from build123d import *

# Parameters (mm, degrees)
BOSS_EXTRUDE1_DEPTH      = 37.5
BOSS_EXTRUDE1_DEPTH_BACK = 37.5
SKETCH1_W                = 20
SKETCH1_H                = 10
SKETCH3_W                = 20
SKETCH3_H                = 5
BOSS_EXTRUDE2_DEPTH      = 20
FILLET1_R                = 10
SKETCH5_W                = 20
SKETCH5_H                = 5
BOSS_EXTRUDE3_DEPTH      = 25
CHAMFER1_SIZE            = 5
CHAMFER1_SIZE_2          = 8.660254038
FILLET2_R                = 10
CUT_EXTRUDE1_DEPTH       = 65.08002809
CUT_EXTRUDE1_DEPTH_BACK  = 65.08002809
SKETCH4_R                = 2.75
CUT_EXTRUDE2_DEPTH       = 66.048059156
CUT_EXTRUDE2_DEPTH_BACK  = 2.5


# Some blends are built 0.0001 mm under size
with BuildPart() as part:
    # Sketch1 → Boss-Extrude1 (new, two sides: drawn at the far end of the back side and taken through both)
    with BuildSketch(Plane.XY.offset(-BOSS_EXTRUDE1_DEPTH_BACK)):
        Rectangle(SKETCH1_W, SKETCH1_H)
    extrude(amount=BOSS_EXTRUDE1_DEPTH + BOSS_EXTRUDE1_DEPTH_BACK)

    # Sketch3 → Boss-Extrude2 (add)
    with BuildSketch(Plane(origin=(0, 0, -37.5), x_dir=(-1, 0, 0), z_dir=(0, 0, -1))):
        Rectangle(SKETCH3_W, SKETCH3_H)
    extrude(amount=BOSS_EXTRUDE2_DEPTH)

    # Fillet1
    fillet1_edges = [part.edges().sort_by_distance(p)[0] for p in [
        (-10, 0, -57.5),
        (10, 0, -57.5),
    ]]
    fillet(fillet1_edges, radius=FILLET1_R - 0.0001)  # a hair under: the kernel refuses the full size

    # Sketch5 → Boss-Extrude3 (add)
    with BuildSketch(Plane.XY.offset(37.5)):
        with Locations((0, 5)):
            Rectangle(SKETCH5_W, SKETCH5_H)
        with Locations((0, -5)):
            Rectangle(SKETCH5_W, SKETCH5_H)
    extrude(amount=BOSS_EXTRUDE3_DEPTH)

    # Chamfer1
    # the kernel refuses this chamfer: 8.660254038, 5 mm, written as the material it adds along each edge
    with BuildSketch(Plane(origin=(10, 5, 37.5), x_dir=(0, -0.05789386240267149, -0.9983227437537926), z_dir=(-1, 0, 0))) as chamfer1_piece_1_section:
        Polygon((CHAMFER1_SIZE * 0.998322743754, -CHAMFER1_SIZE * 0.0578938624027), (-CHAMFER1_SIZE_2 * 0.0578938624016, -CHAMFER1_SIZE_2 * 0.998322743736), (0, 0), align=None)
    chamfer1_piece_1 = extrude(amount=20, mode=Mode.PRIVATE)
    chamfer1_piece_1 = split(chamfer1_piece_1, bisect_by=Plane(origin=(0, 7.5, 35.327003025), z_dir=(0, -1, 0)), keep=Keep.TOP, mode=Mode.PRIVATE)
    add(chamfer1_piece_1)
    with BuildSketch(Plane(origin=(-10, -5, 37.5), x_dir=(0, 0.05789386240267149, -0.9983227437537926), z_dir=(1, 0, 0))) as chamfer1_piece_2_section:
        Polygon((CHAMFER1_SIZE * 0.998322743754, -CHAMFER1_SIZE * 0.0578938624027), (-CHAMFER1_SIZE_2 * 0.0578938624016, -CHAMFER1_SIZE_2 * 0.998322743736), (0, 0), align=None)
    chamfer1_piece_2 = extrude(amount=20, mode=Mode.PRIVATE)
    chamfer1_piece_2 = split(chamfer1_piece_2, bisect_by=Plane(origin=(0, -7.5, 35.327003025), z_dir=(0, 1, 0)), keep=Keep.TOP, mode=Mode.PRIVATE)
    add(chamfer1_piece_2)
    # the kernel refuses this chamfer: 8.660254038, 5 mm, written as the material it takes off along each edge
    with BuildSketch(Plane(origin=(32.404819853, 5, -37.5), x_dir=(0, 0.019326765612700598, 0.9998132206222078), z_dir=(-1, 0, 0))) as chamfer1_2_piece_1_section:
        Polygon((CHAMFER1_SIZE_2 * 0.999813220604, -CHAMFER1_SIZE_2 * 0.0193267656124), (-CHAMFER1_SIZE * 0.0193267656127, -CHAMFER1_SIZE * 0.999813220622), (0, 0), align=None)
    chamfer1_2_piece_1 = extrude(amount=64.809639706, mode=Mode.PRIVATE)
    chamfer1_2_piece_1 = split(chamfer1_2_piece_1, bisect_by=Plane(origin=(0, 2.5, -34.039331058), z_dir=(0, 1, 0)), keep=Keep.TOP, mode=Mode.PRIVATE)
    add(chamfer1_2_piece_1, mode=Mode.SUBTRACT)
    with BuildSketch(Plane(origin=(-32.404819853, -5, -37.5), x_dir=(0, 0.9983227437537926, -0.057893862402671824), z_dir=(1, 0, 0))) as chamfer1_2_piece_2_section:
        Polygon((CHAMFER1_SIZE * 0.998322743754, CHAMFER1_SIZE * 0.0578938624027), (-CHAMFER1_SIZE_2 * 0.0578938624016, CHAMFER1_SIZE_2 * 0.998322743736), (0, 0), align=None)
    chamfer1_2_piece_2 = extrude(amount=64.809639706, mode=Mode.PRIVATE)
    chamfer1_2_piece_2 = split(chamfer1_2_piece_2, bisect_by=Plane(origin=(0, -2.5, -34.039331058), z_dir=(0, -1, 0)), keep=Keep.TOP, mode=Mode.PRIVATE)
    add(chamfer1_2_piece_2, mode=Mode.SUBTRACT)

    # Fillet2
    fillet2_edges = [part.edges().sort_by_distance(p)[0] for p in [
        (-10, -5, 62.5),
        (-10, 5, 62.5),
        (10, -5, 62.5),
        (10, 5, 62.5),
    ]]
    fillet(fillet2_edges, radius=FILLET2_R - 0.0001)  # a hair under: the kernel refuses the full size

    # Sketch4 → Cut-Extrude1 (cut, two sides: drawn at the far end of the back side and taken through both)
    with BuildSketch(Plane(origin=(0, 2.5, 0), x_dir=(1, 0, 0), z_dir=(0, 1, 0)).offset(-CUT_EXTRUDE1_DEPTH_BACK)):
        with Locations(Location((0, 47.5, 0), (0, 0, 270))):
            Circle(SKETCH4_R)
        with Locations(Location((0, -52.5, 0), (0, 0, 270))):
            Circle(SKETCH4_R)
    extrude(amount=CUT_EXTRUDE1_DEPTH + CUT_EXTRUDE1_DEPTH_BACK, mode=Mode.SUBTRACT)

    # Sketch6 → Cut-Extrude2 (cut, two sides: drawn at the far end of the back side and taken through both)
    with BuildSketch(Plane(origin=(0, 7.5, 0), x_dir=(1, 0, 0), z_dir=(0, 1, 0)).offset(-CUT_EXTRUDE2_DEPTH_BACK)):
        Polygon((-2.38156986, -48.375), (-4.763139721, -52.5), (-2.38156986, -56.625), (2.38156986, -56.625), (4.763139721, -52.5), (2.38156986, -48.375), align=None)
    extrude(amount=CUT_EXTRUDE2_DEPTH + CUT_EXTRUDE2_DEPTH_BACK, mode=Mode.SUBTRACT)


solid = part.part
Source: CAD feature listing. Evaluate the final solid. Frame: model axes, mm. A direction names the side the tool comes from. Give positions to 0.01 mm unless a question says otherwise; leave off trailing zeros. Order: outer loops, then holes, each group sorted by start corner. A loop starts at its lowest first (then second) coordinate and runs counter-clockwise, first axis right, second up. Notation, with made-up numbers: (3, 86.25) -> (27, 86.25) arc R31 cw to (27, 116.25) -> close; hole circle Ø1 at (-18.5, 44.5). An arc over 180 degrees is marked (long way). Write item = value, one per line.
Item 1: Section query C-C (x = -7.25). Output: boundary loops of the cut face in (y, z), then the cut area to 3 significant figures.
Check result:
outline = (-7.5, 33.94) -> (-5, 32.5) -> (-5, -28.84) -> (-2.5, -33.17) -> (-2.5, -54.39) -> (2.5, -54.39) -> (2.5, -33.17) -> (5, -28.84) -> (5, 32.5) -> (7.5, 33.94) -> (7.5, 59.39) -> (2.5, 59.39) -> (2.5, 37.5) -> (-2.5, 37.5) -> (-2.5, 59.39) -> (-7.5, 59.39) -> close
area = 1,040 mm²
Item 2: Mould query, pull axis Z, two halves, no side actions, for faces 4 (the face through (-0.14, -6.23, 33.21)), 5 (the face through (0, -2.5, 47)), 6 (the face through (1, 5, 49.7)). Classes: +Z half, -Z half, draft (parallel to the pull), parting line (faces both ways), or undercut.
Check result:
face_4 = -Z half
face_5 = draft
face_6 = undercut
Item 3: Section query B-B (z = 54). Output: boundary loops of the cut face in (x, y).
Check result:
outline = (-9.89, -7.5) -> (-2.3, -7.5) -> (-2.3, -2.5) -> (-9.89, -2.5) -> close; (-9.89, 2.5) -> (-2.3, 2.5) -> (-2.3, 5) -> (-3.9, 5) -> (-3.9, 7.5) -> (-9.89, 7.5) -> close; (2.3, -7.5) -> (9.89, -7.5) -> (9.89, -2.5) -> (2.3, -2.5) -> close; (2.3, 2.5) -> (9.89, 2.5) -> (9.89, 7.5) -> (3.9, 7.5) -> (3.9, 5) -> (2.3, 5) -> close
Item 4: Section query D-D (z = -36). Output: boundary loops of the cut face in (x, y).
Check result:
outline = (-10, -2.5) -> (10, -2.5) -> (10, 2.5) -> (-10, 2.5) -> close
Item 5: Contact query for flat-ended pins moving along their axis: pin 1 (6 mm diameter, centred on x = -0.5, z = -40.5, fed in from +Y); pin 2 (1 mm diameter, centred on x = -5, y = 1.5, fed in from -Z); pin 3 (2 mm diameter, centred on x = 1, y = -5, fed in from -Z); pin 4 (4.5 mm diameter, centred on x = 0, z = -47.5, fed in from +Y). Output: stop coordinate, or through.
Check result:
pin_1 = 2.5
pin_2 = -56.43
pin_3 = -30.57
pin_4 = through
Item 6: Ray query, probe 1 along Z at (x, y) = (0, 0.95); probe 2 along Y at (x, z) = (-0.5, 46.5); probe 3 along X at (y, z) = (-5.1, 52.5). Return the intervals inside material, ascending.
Check result:
probe_1 = -57.5 to -50.25, -44.75 to 37.5
probe_2 = -7.5 to -2.5, 2.5 to 7.5
probe_3 = -10 to -2.75, 2.75 to 10
Item 7: Set-up query: faces 1 (the face through (0, -5, 1)), 2 (the face through (0, 2.5, -42)), 3 (the face through (0, 6, 56.625)). Return all of +Z, -Z, +X, -X, +Y, -Y with unobstructed straight access to the full face (end or side cutting, diameter ignored); none if empty.
Check result:
face_1 = -Z, +X, -X, -Y
face_2 = -Z, +X, -X, +Y
face_3 = +Y
